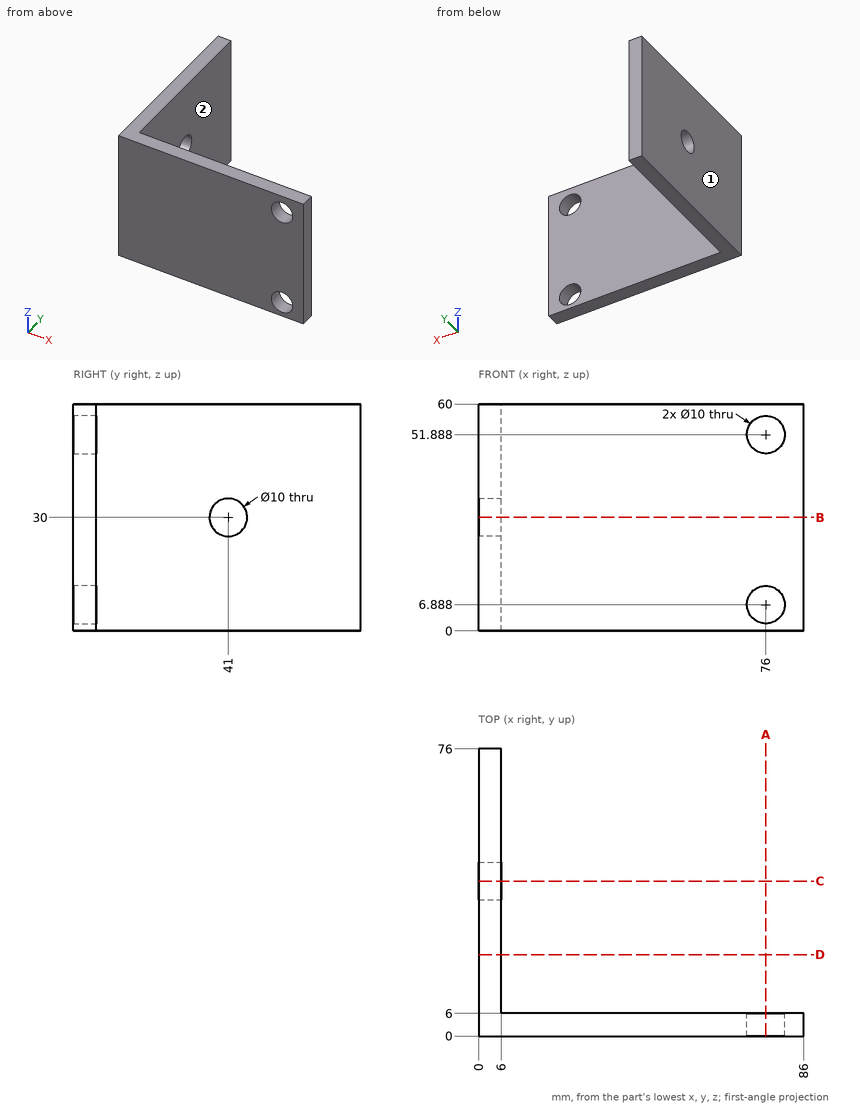
For this review, use the dimensioned drawing (mm, ordinates from the lowest corner) and the shaded views. A direction names the side the tool comes from. Round coordinates to 2 decimals unless told otherwise and drop trailing zeros. Write each loop counter-clockwise with the first axis right and the second up, starting at its lowest first coordinate (ties: lowest second). Pieces come first, ordered by that corner, then holes. Notation, with made-up numbers: (25, 83) -> (67, 83) arc R13 ccw to (67, 106) -> close; hole circle Ø6 at (69, 52.5). An arc over 180 degrees is marked (long way). Use CSV: the item, a comma, the result in double quotes.
(1) Consider section C-C, the plane y = 41. Give the boundary of the cut face in (x, z).
Computed values:
outline,"(0, 0) -> (6, 0) -> (6, 25) -> (0, 25) -> close; (0, 35) -> (6, 35) -> (6, 60) -> (0, 60) -> close"
(2) Clearance check with flat-ended pins moving along their axes: P1, Ø2, axis at x = 27, z = 11, coming from the +Y side; P2, Ø18, axis at y = 35, z = 26.5, coming from the +X side. State where each tip first meets the part, or that it passes through.
Computed values:
P1,"y = 6"
P2,"x = 6"
(3) Consider section B-B, the plane z = 30. Give the boundary of the cut face in (x, y).
Computed values:
outline,"(0, 0) -> (86, 0) -> (86, 6) -> (6, 6) -> (6, 36) -> (0, 36) -> close; (0, 46) -> (6, 46) -> (6, 76) -> (0, 76) -> close"
(4) For the marked faces 1 and 2, list the 3-axis set-ups (+Z, -Z, +X, -X, +Y, -Y) from which the entire face can be reached by the end or side of a thin tool; tool diameter is ignored.
Computed values:
face 1,"+Z, -Z, -X, +Y, -Y"
face 2,"+Z, -Z, +X, +Y"
(5) Consider section D-D, the plane y = 21.5. Give the boundary of the cut face in (x, z).
Computed values:
outline,"(0, 0) -> (6, 0) -> (6, 60) -> (0, 60) -> close"
(6) To check wall thickness, follow L1, parallel to X at y = 35.5, z = 50; L2, parallel to Y at x = 4.6, z = 30. State the ranges of each line that lie inside material, in increasing order. Write a range as [from, to].
Computed values:
L1,"[0, 6]"
L2,"[0, 36], [46, 76]"
(7) Consider section A-A, the plane x = 76. Give the boundary of the cut face in (y, z).
Computed values:
outline,"(0, 0) -> (6, 0) -> (6, 1.89) -> (0, 1.89) -> close; (0, 11.89) -> (6, 11.89) -> (6, 46.89) -> (0, 46.89) -> close; (0, 56.89) -> (6, 56.89) -> (6, 60) -> (0, 60) -> close"
